Study the drawing (mm; zero at the part's minimum x, y, z) and answer. Coordinates: 2 decimals unless noted, no trailing zeros. Order: outer loops, then holes, each group sorted by start corner. A loop starts at its lowest first (then second) coordinate and runs counter-clockwise, first axis right, second up.
1. Flat-ended cylindrical pins translate along their axes: pin 1 Ø3 at (x, y) = (135.5, 50) entering from -Z; pin 2 Ø0.9 at (x, z) = (172.5, 1.5) entering from -Y. Find the tip coordinate at first contact, or state that the pin passes through.
2. The part is cut by section A-A, the plane z = 1.9. Give the vertices of the cut face in (x, y).
3. The part is cut by section B-B, the plane x = 169. Give the vertices of the cut face in (y, z), then the cut area to 3 significant figures.
4. Find the intervals of material crossed by probe 1 along X at (y, z) = (26, 0.9); probe 2 along Y at (x, z) = (187.5, 0.25), in increasing order.
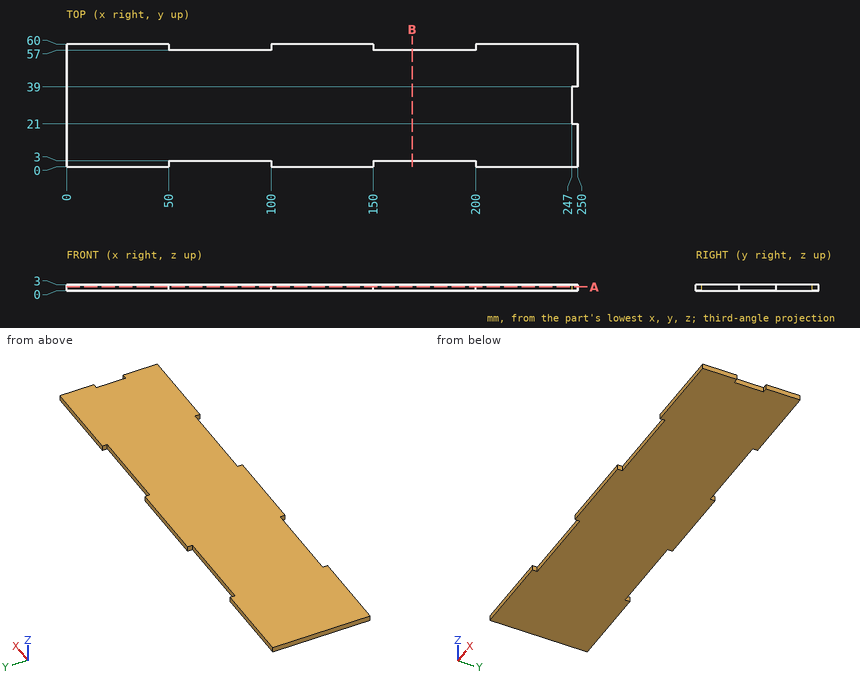
Geometry says:
1. pin 1: stops at z = 0
1. pin 2: stops at y = 3
2. outline: (0, 0) - (50, 0) - (50, 3) - (100, 3) - (100, 0) - (150, 0) - (150, 3) - (200, 3) - (200, 0) - (250, 0) - (250, 21) - (247, 21) - (247, 39) - (250, 39) - (250, 60) - (200, 60) - (200, 57) - (150, 57) - (150, 60) - (100, 60) - (100, 57) - (50, 57) - (50, 60) - (0, 60) - close
3. outline: (3, 0) - (57, 0) - (57, 3) - (3, 3) - close
3. area: 162 mm2
4. probe 1: x = 0 to 247
4. probe 2: y = 3 to 57
